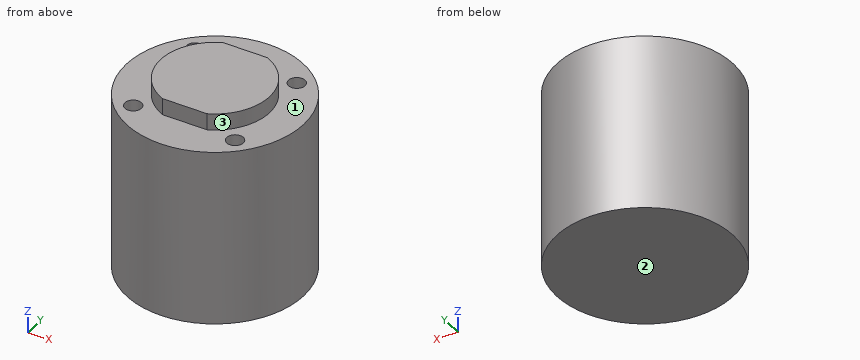
from build123d import *

# Parameters (mm, degrees)
BOSS_EXTRUDE1_DEPTH = 3
SKETCH2_R           = 16
BOSS_EXTRUDE2_DEPTH = 32
SKETCH6_R           = 1.5
CUT_EXTRUDE1_DEPTH  = 10


with BuildPart() as part:
    # Sketch1 → Boss-Extrude1 (new body)
    with BuildSketch(Plane.XY):
        with BuildLine():
            Line((-4.002811512, 9), (4.002811512, 9))
            ThreePointArc((4.002811512, 9), (9.85, 0), (4.002811512, -9))
            Line((4.002811512, -9), (-4.002811512, -9))
            ThreePointArc((-4.002811512, -9), (-9.85, 0), (-4.002811512, 9))
        make_face()
    extrude(amount=BOSS_EXTRUDE1_DEPTH)

    # Sketch2 → Boss-Extrude2 (add)
    with BuildSketch(Plane(origin=(0, 0, 0), x_dir=(-1, 0, 0), z_dir=(0, 0, -1))):
        Circle(SKETCH2_R)
    extrude(amount=BOSS_EXTRUDE2_DEPTH)

    # Sketch6 → Cut-Extrude1 (cut)
    with BuildSketch(Plane.XY):
        with Locations((-9.192388155, 9.192388155)):
            Circle(SKETCH6_R)
        with Locations((9.192388155, 9.192388155)):
            Circle(SKETCH6_R)
        with Locations((9.192388155, -9.192388155)):
            Circle(SKETCH6_R)
        with Locations((-9.192388155, -9.192388155)):
            Circle(SKETCH6_R)
    extrude(amount=-CUT_EXTRUDE1_DEPTH, mode=Mode.SUBTRACT)


solid = part.part
Read the model definition and answer for the solid it produces. Units are mm, in the model's axes. Face numbers are marked on the shaded views. A direction names the side the tool comes from. Coordinates: 2 decimals unless noted, no trailing zeros. Loops run counter-clockwise (first coordinate to the right, second up) from the corner with the lowest first, then second, coordinate; pieces in that order, holes last. Notation, with made-up numbers: (16, 71) -> (43, 71) arc R17 ccw to (43, 104) -> close; hole circle Ø10 at (-14.75, -21.5). An arc over 180 degrees is marked (long way). Write item = value, one per line. Start each with the question number.
1) For the marked faces 1, 2 and 3, determine the directions among +Z, -Z, +X, -X, +Y, -Y from which every point of the face is accessible in a straight line to the end or side of a thin tool.
2) Given P1, Ø8, axis at y = -5, z = -20.5, coming from the -X side; P2, Ø1, axis at x = 1.5, z = -3.5, coming from the +Y side; P3, Ø3.5, axis at x = -10, y = -10, coming from the +Z side, each flat-ended and moving along its own axis, determine where each tip first touches the part or whether it passes through.
3) The part is cut by section D-D, the plane z = -14.5. Determine the outline of the cut face in (x, y).
4) Find the intervals of material crossed by L1, parallel to X at y = 8, z = -3; L2, parallel to Z at x = 8, y = -11.5; L3, parallel to Y at x = 0, z = -10.5, in increasing order. Write a range as from..to.
5) The part is cut by section C-C, the plane z = -8. Determine the outline of the cut face in (x, y), plus the area to 3 significant figures.
6) The part is cut by section B-B, the plane y = 0. Determine the outline of the cut face in (x, z).
7) The part is cut by section A-A, the plane x = 0. Determine the outline of the cut face in (y, z).
Result:
q1.face_1 = +Z
q1.face_2 = -Z, +X, -X, +Y, -Y
q1.face_3 = +Z, +X
q2.P1 = -15.97
q2.P2 = 15.97
q2.P3 = 0
q3.outline = circle Ø32 at (0, 0)
q4.L1 = -13.86..-10.1, -8.28..8.28, 10.1..13.86
q4.L2 = -32..0
q4.L3 = -16..16
q5.outline = circle Ø32 at (0, 0); hole circle Ø3 at (-9.19, -9.19); hole circle Ø3 at (-9.19, 9.19); hole circle Ø3 at (9.19, -9.19); hole circle Ø3 at (9.19, 9.19)
q5.area = 776 mm²
q6.outline = (-16, -32) -> (16, -32) -> (16, 0) -> (9.85, 0) -> (9.85, 3) -> (-9.85, 3) -> (-9.85, 0) -> (-16, 0) -> close
q7.outline = (-16, -32) -> (16, -32) -> (16, 0) -> (9, 0) -> (9, 3) -> (-9, 3) -> (-9, 0) -> (-16, 0) -> close
